Can you work these out from the model? Positions are in its coordinate system, mm. Face numbers are marked on the shaded views. A direction names the side the tool comes from. Round coordinates to 2 decimals unless told otherwise and drop trailing zeros. Write each loop counter-clockwise with the first axis right and the second up, starting at its lowest first coordinate (ties: lowest second). Pieces come first, ordered by that corner, then holes. Notation, with made-up numbers: M 15.25,-4 L 34.25,-4 A8 cw 34.25,3 Z; hole C -28,7.25 d9. An arc over 180 degrees is marked long. Use one line per item in the form item = value. Start each with the question number.
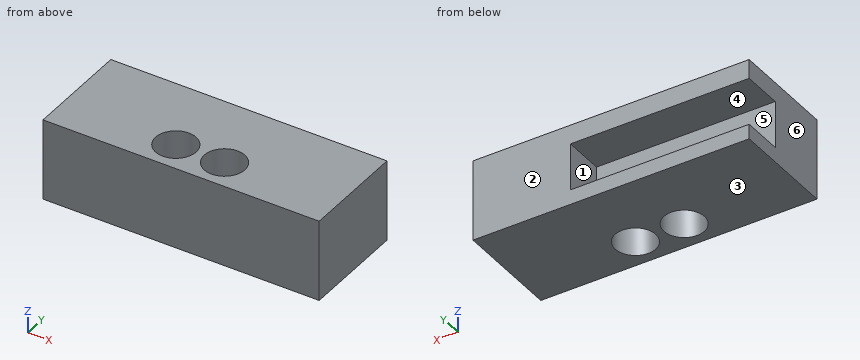
```python
from build123d import *

# Parameters (mm, degrees)
SKETCH_1_W          = 34
SKETCH_1_H          = 10
EXTRUDE_2_DEPTH     = 13
SKETCH_2_W          = 22
SKETCH_2_H          = 5.8
CUT_EXTRUDE_1_DEPTH = 5
SKETCH_3_R          = 2.5
CUT_EXTRUDE_2_DEPTH = 20


with BuildPart() as part:
    # 草圖1 → 填料-伸長2 (new body)
    with BuildSketch(Plane(origin=(0, 0, 0), x_dir=(1, 0, 0), z_dir=(0, 1, 0))):
        with Locations((0.708333333, 1.1625)):
            Rectangle(SKETCH_1_W, SKETCH_1_H)
    extrude(amount=EXTRUDE_2_DEPTH)

    # 草圖2 → 除料-伸長1 (cut)
    with BuildSketch(Plane(origin=(0, 13, 0), x_dir=(1, 0, 0), z_dir=(0, 1, 0))):
        with Locations((-5.291666667, 1.430875321)):
            Rectangle(SKETCH_2_W, SKETCH_2_H)
    extrude(amount=-CUT_EXTRUDE_1_DEPTH, mode=Mode.SUBTRACT)

    # 草圖3 → 除料-伸長2 (cut)
    with BuildSketch(Plane(origin=(0, 0, -6.1625), x_dir=(-1, 0, 0), z_dir=(0, 0, -1))):
        with Locations((2.291666667, 3.663194133)):
            Circle(SKETCH_3_R)
        with Locations((-3.708333333, 3.663194133)):
            Circle(SKETCH_3_R)
    extrude(amount=-CUT_EXTRUDE_2_DEPTH, mode=Mode.SUBTRACT)


solid = part.part
```
1. If we section it at B-B (y = 5.75): List the corners of the cut face in (x, z) for me, and give its area (3 significant figures).
2. Please list where these lines run through material, in increasing order: line 1 along X through (y, z) = (3, -5); line 2 along X through (y, z) = (2.75, -5.25); line 3 along Y through (x, z) = (-9.5, -0.5).
3. If we section it at D-D (y = 8.5): List the corners of the cut face in (x, z) for me, and give its area (3 significant figures).
4. Which directions (+Z, -Z, +X, -X, +Y, -Y) give clear straight access to the entire face, cutting with the end or side of a thin tool? Please do the marked faces 1 and 2.
5. If we section it at A-A (x = -2.5): List the corners of the cut face in (y, z) for me.
6. If we mould it in two halves opening along Z, with no side actions, what happens to the marked faces 3, 4, 5 and 6? For each: pulls with the +Z half, pulls with the -Z half, needs draft (parallel to the pull), parting line crosses it, or undercut.
7. Will these pins go through, and if not, where does the flat tip stop? pin 1 (1 mm diameter, centred on x = -4, z = -1.5, fed in from +Y); pin 2 (1.5 mm diameter, centred on y = 10.5, z = -2.5, fed in from -X).
8. If we section it at C-C (z = -3.75): List the corners of the cut face in (x, y) for me, and give its area (3 significant figures).
Model answer:
q1.outline = M -16.29,-6.16 L -3.67,-6.16 L -3.67,3.84 L -16.29,3.84 Z; M -0.91,-6.16 L 2.33,-6.16 L 2.33,3.84 L -0.91,3.84 Z; M 5.09,-6.16 L 17.71,-6.16 L 17.71,3.84 L 5.09,3.84 Z
q1.area = 285 mm2
q2.line_1 = -16.29 to -4.7, 0.12 to 1.3, 6.12 to 17.71
q2.line_2 = -16.29 to -4.62, 0.04 to 1.38, 6.04 to 17.71
q2.line_3 = 0 to 8
q3.outline = M -16.29,-6.16 L 17.71,-6.16 L 17.71,3.84 L -16.29,3.84 L -16.29,1.47 L 5.71,1.47 L 5.71,-4.33 L -16.29,-4.33 Z
q3.area = 212 mm2
q4.face_1 = -X, +Y
q4.face_2 = +Z, -Z, +X, -X, +Y
q5.outline = M 0,-6.16 L 1.17,-6.16 L 1.17,3.84 L 0,3.84 Z; M 6.15,-6.16 L 13,-6.16 L 13,-4.33 L 8,-4.33 L 8,1.47 L 13,1.47 L 13,3.84 L 6.15,3.84 Z
q6.face_3 = pulls with the -Z half
q6.face_4 = undercut
q6.face_5 = undercut
q6.face_6 = needs draft
q7.pin_1 = 8
q7.pin_2 = 5.71
q8.outline = M -16.29,0 L 17.71,0 L 17.71,13 L 5.71,13 L 5.71,8 L -16.29,8 Z; hole C -2.29,3.66 d5; hole C 3.71,3.66 d5
q8.area = 293 mm2
